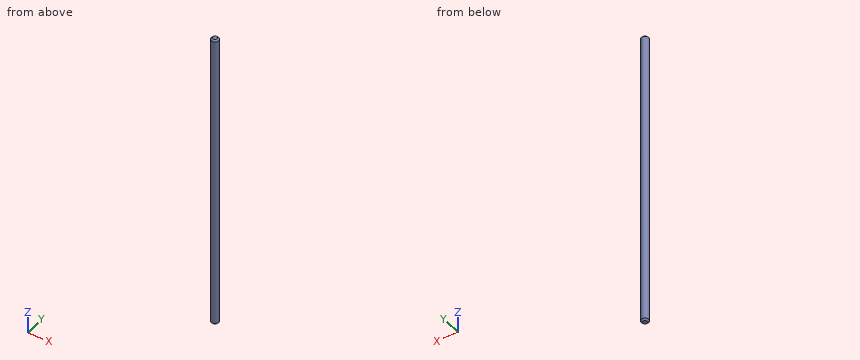
Autodesk Inventor part; units mm, degrees
ref_plane "YZ Plane" through (0, 0, 0) normal (1, 0, 0) x (0, 1, 0)
ref_plane "XZ Plane" through (0, 0, 0) normal (0, 1, 0) x (-1, 0, 0)
ref_plane "XY Plane" through (0, 0, 0) normal (0, 0, 1) x (1, 0, 0)
sketch "Skizze1" plane through (0, 0, 0) normal (0, 1, 0) x (-1, 0, 0)
  line L0 (0, 0) -> (5, 0)
  line L1 (5, 0) -> (5, -200)
  line L2 (5, -200) -> (0, -200)
  line L3 (0, -200) -> (0, 0)
  dimension "d0" = 200
  dimension "d1" = 10
revolve "Umdrehung1" add sketch "Skizze1" angle 360 about axis through (0, 0, -200) along (0, 0, 1)
thread "Gewinde1"
chamfer "Fase1" distance 2 angle 45 1 edges at (5, 0, 0)
mirror "Spiegeln1" about plane through (0, 0, -200) normal (0, 0, -1)
properties part number "Gewindestange" material "Stahl AISI 4130"
Could you check a few things on this model? Use its own coordinates, in mm. Coordinates: 2 decimals unless noted, no trailing zeros. Write each loop counter-clockwise with the first axis right and the second up, starting at its lowest first coordinate (ties: lowest second). Pieces come first, ordered by that corner, then holes. Notation, with made-up numbers: (39.25, 44) -> (72.25, 44) arc R18 ccw to (72.25, 73) -> close; hole circle Ø3 at (-36, 67). An arc over 180 degrees is marked (long way). Write item = value, one per line. Start each with the question number.
(1) Will this pin go through, and if not, where does the flat tip stop? pin 1 (1 mm diameter, centred on x = 1, z = -342.5, fed in from -Y).
(2) I want a section at A-A (z = -111). Please give me the cut outline in (x, y), plus the area to 3 significant figures.
(3) I need wall thicknesses on line 1 (Y direction, x = 0.5, z = -219.5); line 2 (Y direction, x = -4, z = -136). Which ranges of each line are inside material? Lowest first, please. Write a range as [from, to].
Result set:
q1.pin_1 = -4.97
q2.outline = circle Ø10 at (0, 0)
q2.area = 78.5 mm2
q3.line_1 = [-4.97, 4.97]
q3.line_2 = [-3, 3]
